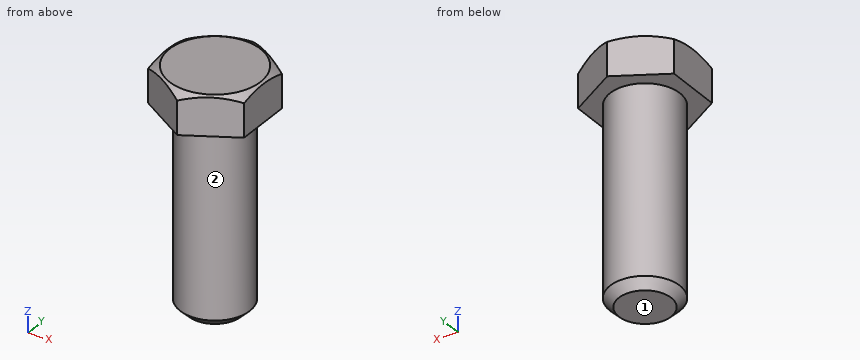
from build123d import *

# Parameters (mm, degrees)
EXTRUDE_337_DEPTH     = 9
SKETCH_D_OUTSIDE_W    = 65.598
SKETCH_D_OUTSIDE_H    = 69.002
SKETCH_D_OUTSIDE_R    = 10.45
CUT_EXTRUDE_379_DEPTH = 10
CUT_EXTRUDE_379_DRAFT = -60
SKETCH_398_R          = 8
EXTRUDE_460_DEPTH     = 45
CHAMFER_475_SIZE      = 2


with BuildPart() as part:
    # Sketch 332 → Extrude 337 (new body)
    with BuildSketch(Plane.XY):
        Polygon((0, -12.701705922), (11, -6.350852961), (11, 6.350852961), (0, 12.701705922), (-11, 6.350852961), (-11, -6.350852961), align=None)
    extrude(amount=EXTRUDE_337_DEPTH)


with BuildPart() as cut_extrude_379_tool:
    # D outside → Cut-Extrude 379 (with draft: the straight prism first)
    with BuildSketch(Plane.XY.offset(9)):
        Rectangle(SKETCH_D_OUTSIDE_W, SKETCH_D_OUTSIDE_H)
        Circle(SKETCH_D_OUTSIDE_R, mode=Mode.SUBTRACT)
    extrude(amount=-CUT_EXTRUDE_379_DEPTH)
    # Cut-Extrude 379: the draft: its side faces are tilted about the plane it starts from
    cut_extrude_379_sides = [cut_extrude_379_tool.faces().sort_by_distance(p)[0] for p in [
        (0, -34.501, 4),
        (32.799, 0, 4),
        (0, 34.501, 4),
        (-32.799, 0, 4),
        (-10.45, 0, 4),
    ]]
    draft(cut_extrude_379_sides, Plane.XY.offset(9), CUT_EXTRUDE_379_DRAFT)


with BuildPart() as part_1:
    add(part.part)

    # Cut-Extrude 379: cut by cut_extrude_379_tool
    add(cut_extrude_379_tool.part, mode=Mode.SUBTRACT)

    # Sketch 398 → Extrude 460 (add)
    with BuildSketch(Plane(origin=(0, 0, 0), x_dir=(-1, 0, 0), z_dir=(0, 0, -1))):
        with Locations(Location((0, 0, 0), (0, 0, 180))):
            Circle(SKETCH_398_R)
    extrude(amount=EXTRUDE_460_DEPTH)

    # Chamfer 475
    chamfer_475_edges = [part_1.edges().sort_by_distance(p)[0] for p in [
        (-8, 0, -45),
    ]]
    chamfer(chamfer_475_edges, length=CHAMFER_475_SIZE)


solid = part_1.part
For this review, take the finished solid that the model builds, in its own axes (mm). Face numbers are marked on the shaded views. A direction names the side the tool comes from. Round coordinates to 2 decimals unless told otherwise and drop trailing zeros. Loops run counter-clockwise (first coordinate to the right, second up) from the corner with the lowest first, then second, coordinate; pieces in that order, holes last. Notation, with made-up numbers: (24.25, 49) - (72.25, 49) arc R30 cw to (72.25, 85) - close; hole circle Ø11 at (29, -13). An arc over 180 degrees is marked (long way). Use one line per item in the form item = value.
1) Clearance check with flat-ended pins moving along their axes: P1, Ø4, axis at y = 6, z = -37, coming from the +X side; P2, Ø2, axis at x = -3, z = 0.5, coming from the +Y side; P3, Ø1.5, axis at y = 0, z = -3, coming from the -X side. State where each tip first meets the part, or that it passes through.
Solutions:
P1 = 6.93
P2 = 11.55
P3 = -8
2) We need section A-A on z = 4.5. Write out the cut boundary in (x, y).
Solutions:
outline = (-11, -6.35) - (0, -12.7) - (11, -6.35) - (11, 6.35) - (0, 12.7) - (-11, 6.35) - close
3) We need section C-C on z = -18. Write out the cut boundary in (x, y).
Solutions:
outline = circle Ø16 at (0, 0)
4) We need section B-B on y = 0. Write out the cut boundary in (x, z).
Solutions:
outline = (-11, 0) - (-8, 0) - (-8, -43) - (-6, -45) - (6, -45) - (8, -43) - (8, 0) - (11, 0) - (11, 8.68) - (10.45, 9) - (-10.45, 9) - (-11, 8.68) - close
5) Tool access review of the marked faces 1 and 2: name each direction out of +Z, -Z, +X, -X, +Y, -Y from which nothing blocks a thin tool from reaching the whole face with its end or side.
Solutions:
face_1 = -Z, +X, -X, +Y, -Y
face_2 = -Z
6) Wall thickness on probe 1 along Z at (x, y) = (9.75, -3); probe 2 along Y at (x, z) = (-2.25, 1); probe 3 along Y at (x, z) = (2.25, -27.5): over which ranges is each line inside the solid? List them lowest first.
Solutions:
probe_1 = 0 to 9
probe_2 = -11.4 to 11.4
probe_3 = -7.68 to 7.68
